Source: CAD feature listing. Evaluate the final solid. Frame: model axes, mm. A direction names the side the tool comes from. Give positions to 0.01 mm unless a question says otherwise; leave off trailing zeros. Write each loop counter-clockwise with the first axis right and the second up, starting at its lowest first coordinate (ties: lowest second). Pieces come first, ordered by that corner, then holes. Notation, with made-up numbers: (34, -36) - (73, -36) arc R17 ccw to (73, -22) - close; hole circle Ø11 at (20, 40.25). An arc over 180 degrees is marked (long way). Answer as a JSON object with one key per item and string values. Group by question number.
from build123d import *

# Parameters (mm, degrees)
EXTRUDE_1_DEPTH     = 6
SKETCH_3_R          = 1.4
CUT_EXTRUDE_1_DEPTH = 6
SKETCH_4_R          = 5
EXTRUDE_2_DEPTH     = 12
CUT_EXTRUDE_2_DEPTH = 12
SKETCH_6_R          = 1.5
CUT_EXTRUDE_3_DEPTH = 31
SKETCH_7_R          = 1.5
SKETCH_7_R_2        = 1.4
EXTRUDE_3_DEPTH     = 18
CUT_EXTRUDE_4_DEPTH = 3


with BuildPart() as part:
    # 草图2 → 凸台-拉伸1 (new body)
    with BuildSketch(Plane(origin=(0, 0, 0), x_dir=(1, 0, 0), z_dir=(0, 1, 0))):
        with BuildLine():
            Line((-1.1, 10.341663309), (-1.3, 12.432216214))
            ThreePointArc((-1.3, 12.432216214), (0, 12.5), (1.3, 12.432216214))
            Line((1.3, 12.432216214), (1.1, 10.341663309))
            ThreePointArc((1.1, 10.341663309), (2.691718069, 10.045628593), (4.21820371, 9.506143143))
            Line((4.21820371, 9.506143143), (5.090275082, 11.416615067))
            ThreePointArc((5.090275082, 11.416615067), (6.25, 10.825317547), (7.341941132, 10.116615067))
            Line((7.341941132, 10.116615067), (6.123459599, 8.406143143))
            ThreePointArc((6.123459599, 8.406143143), (7.353910524, 7.353910524), (8.406143143, 6.123459599))
            Line((8.406143143, 6.123459599), (10.116615067, 7.341941132))
            ThreePointArc((10.116615067, 7.341941132), (10.825317547, 6.25), (11.416615067, 5.090275082))
            Line((11.416615067, 5.090275082), (9.506143143, 4.21820371))
            ThreePointArc((9.506143143, 4.21820371), (10.045628593, 2.691718069), (10.341663309, 1.1))
            Line((10.341663309, 1.1), (12.432216214, 1.3))
            ThreePointArc((12.432216214, 1.3), (12.5, 0), (12.432216214, -1.3))
            Line((12.432216214, -1.3), (10.341663309, -1.1))
            ThreePointArc((10.341663309, -1.1), (10.045628593, -2.691718069), (9.506143143, -4.21820371))
            Line((9.506143143, -4.21820371), (11.416615067, -5.090275082))
            ThreePointArc((11.416615067, -5.090275082), (10.825317547, -6.25), (10.116615067, -7.341941132))
            Line((10.116615067, -7.341941132), (8.406143143, -6.123459599))
            ThreePointArc((8.406143143, -6.123459599), (7.353910524, -7.353910524), (6.123459599, -8.406143143))
            Line((6.123459599, -8.406143143), (7.341941132, -10.116615067))
            ThreePointArc((7.341941132, -10.116615067), (6.25, -10.825317547), (5.090275082, -11.416615067))
            Line((5.090275082, -11.416615067), (4.21820371, -9.506143143))
            ThreePointArc((4.21820371, -9.506143143), (2.691718069, -10.045628593), (1.1, -10.341663309))
            Line((1.1, -10.341663309), (1.3, -12.432216214))
            ThreePointArc((1.3, -12.432216214), (0, -12.5), (-1.3, -12.432216214))
            Line((-1.3, -12.432216214), (-1.1, -10.341663309))
            ThreePointArc((-1.1, -10.341663309), (-2.691718069, -10.045628593), (-4.21820371, -9.506143143))
            Line((-4.21820371, -9.506143143), (-5.090275082, -11.416615067))
            ThreePointArc((-5.090275082, -11.416615067), (-6.25, -10.825317547), (-7.341941132, -10.116615067))
            Line((-7.341941132, -10.116615067), (-6.123459599, -8.406143143))
            ThreePointArc((-6.123459599, -8.406143143), (-7.353910524, -7.353910524), (-8.406143143, -6.123459599))
            Line((-8.406143143, -6.123459599), (-10.116615067, -7.341941132))
            ThreePointArc((-10.116615067, -7.341941132), (-10.825317547, -6.25), (-11.416615067, -5.090275082))
            Line((-11.416615067, -5.090275082), (-9.506143143, -4.21820371))
            ThreePointArc((-9.506143143, -4.21820371), (-10.045628593, -2.691718069), (-10.341663309, -1.1))
            Line((-10.341663309, -1.1), (-12.432216214, -1.3))
            ThreePointArc((-12.432216214, -1.3), (-12.5, 0), (-12.432216214, 1.3))
            Line((-12.432216214, 1.3), (-10.341663309, 1.1))
            ThreePointArc((-10.341663309, 1.1), (-10.045628593, 2.691718069), (-9.506143143, 4.21820371))
            Line((-9.506143143, 4.21820371), (-11.416615067, 5.090275082))
            ThreePointArc((-11.416615067, 5.090275082), (-10.825317547, 6.25), (-10.116615067, 7.341941132))
            Line((-10.116615067, 7.341941132), (-8.406143143, 6.123459599))
            ThreePointArc((-8.406143143, 6.123459599), (-7.353910524, 7.353910524), (-6.123459599, 8.406143143))
            Line((-6.123459599, 8.406143143), (-7.341941132, 10.116615067))
            ThreePointArc((-7.341941132, 10.116615067), (-6.25, 10.825317547), (-5.090275082, 11.416615067))
            Line((-5.090275082, 11.416615067), (-4.21820371, 9.506143143))
            ThreePointArc((-4.21820371, 9.506143143), (-2.691718069, 10.045628593), (-1.1, 10.341663309))
        make_face()
    extrude(amount=EXTRUDE_1_DEPTH)

    # 草图3 → 切除-拉伸1 (cut)
    with BuildSketch(Plane(origin=(0, 6, 0), x_dir=(1, 0, 0), z_dir=(0, 1, 0))):
        with Locations(Location((0, 0, 0), (0, 0, 270))):
            Circle(SKETCH_3_R)
    extrude(amount=-CUT_EXTRUDE_1_DEPTH, mode=Mode.SUBTRACT)

    # 草图4 → 凸台-拉伸2 (add)
    with BuildSketch(Plane(origin=(0, 6, 0), x_dir=(1, 0, 0), z_dir=(0, 1, 0))):
        with Locations(Location((0, 0, 0), (0, 0, 270))):
            Circle(SKETCH_4_R)
    extrude(amount=EXTRUDE_2_DEPTH)

    # 草图5 → 切除-拉伸2 (cut)
    with BuildSketch(Plane(origin=(0, 18, 0), x_dir=(1, 0, 0), z_dir=(0, 1, 0))):
        with BuildLine():
            Line((-1, -1.118033989), (1, -1.118033989))
            ThreePointArc((1, -1.118033989), (0, 1.5), (-1, -1.118033989))
        make_face()
    extrude(amount=-CUT_EXTRUDE_2_DEPTH, mode=Mode.SUBTRACT)

    # 草图6 → 切除-拉伸3 (cut)
    with BuildSketch(Plane(origin=(0, 18, 0), x_dir=(1, 0, 0), z_dir=(0, 1, 0))):
        with Locations(Location((0, 0, 0), (0, 0, 270))):
            Circle(SKETCH_6_R)
    extrude(amount=-CUT_EXTRUDE_3_DEPTH, mode=Mode.SUBTRACT)

    # 草图7 → 凸台-拉伸3 (add)
    with BuildSketch(Plane(origin=(0, 18, 0), x_dir=(1, 0, 0), z_dir=(0, 1, 0))):
        Circle(SKETCH_7_R)
        with Locations(Location((0, 0, 0), (0, 0, 270))):
            Circle(SKETCH_7_R_2, mode=Mode.SUBTRACT)
    extrude(amount=-EXTRUDE_3_DEPTH)

    # 草图8 → 切除-拉伸4 (cut)
    with BuildSketch(Plane(origin=(0, 18, 0), x_dir=(1, 0, 0), z_dir=(0, 1, 0))):
        Polygon((4.041451884, 0), (2.020725942, 3.5), (-2.020725942, 3.5), (-4.041451884, 0), (-2.020725942, -3.5), (2.020725942, -3.5), align=None)
    extrude(amount=-CUT_EXTRUDE_4_DEPTH, mode=Mode.SUBTRACT)

    # 草图9 → 旋转1 (revolve)
    with BuildSketch(Plane(origin=(0, 0, 0), x_dir=(0, 0, -1), z_dir=(1, 0, 0)), mode=Mode.PRIVATE) as revolve_1_sk:
        with BuildLine():
            Line((5, 6), (12.496216833, 6))
            Line((12.496216833, 6), (12.496216833, 6.5))
            ThreePointArc((12.496216833, 6.5), (11.496216833, 7.5), (12.496216833, 8.5))
            Line((12.496216833, 8.5), (12.496216833, 9))
            Line((12.496216833, 9), (5, 9))
            Line((5, 9), (5, 6))
        make_face()
    revolve(revolve_1_sk.sketch.rotate(Axis((0, 17.668891616, 0), (0, -1, 0)), 180), axis=Axis((0, 17.668891616, 0), (0, -1, 0)))


solid = part.part
Q1. Section D-D on y = 7. Return the cut outline in (x, z).
Q2. Draft query along X for faces 1 (the cylindrical face through (10.816, 2.958, -6.266)), 2 (the flat face through (-1.2, 3, -11.4)), 3 (the cylindrical face through (0, 3, 12.5)). Return one class per face: released by +X, released by -X, zero draft, split by the parting line, or undercut.
Q3. Reachability of faces 4 (the flat face through (4.66, 2.96, 10.47)), 5 (the flat face through (3.045, 16.521, -1.726)), 6 (the flat face through (1.2, 3, 11.4)) from +Z, -Z, +X, -X, +Y, -Y: full face, straight path, thin tool, end or side. Return the list, or none.
Q4. First-contact query: pin 1 Ø1.4 at (x, z) = (-11, -5.5) entering from +Y; pin 2 Ø5 at (y, z) = (9, -7.5) entering from +X; pin 3 Ø3 at (x, y) = (4.5, 15.5) entering from -Z. Flat tips, straight axial feed; report the tip coordinate or a pass-through.
Q5. Ray query, probe 1 along X at (y, z) = (8.75, 0); probe 2 along X at (y, z) = (3.25, -6.5). Return the intervals inside material, ascending. Write a range as [from, to].
Q6. Section A-A on y = 15.5. Return the cut outline in (x, z).
Q7. Section C-C on y = 10. Return the cut outline in (x, z).
Taken from the geometry:
{
 "1": {"outline": "circle Ø23.26 at (0, 0); hole circle Ø2.8 at (0, 0)"},
 "2": {"face 1": "released by +X", "face 2": "undercut", "face 3": "split by the parting line"},
 "3": {"face 4": "+Z, -Y", "face 5": "+Y", "face 6": "-Y"},
 "4": {"pin 1": "stops at y = 9", "pin 2": "stops at x = 11.45", "pin 3": "stops at z = -4"},
 "5": {"probe 1": "x = [-12.5, -1.4], [1.4, 12.5]", "probe 2": "x = [-10.68, -8.93], [-8.12, 8.12], [8.93, 10.68]"},
 "6": {"outline": "circle Ø10 at (0, 0); hole (-4.04, 0) - (-2.02, -3.5) - (2.02, -3.5) - (4.04, 0) - (2.02, 3.5) - (-2.02, 3.5) - close"},
 "7": {"outline": "circle Ø10 at (0, 0); hole circle Ø2.8 at (0, 0)"}
}
